Verification items for the finished model (mm, model axes). A direction names the side the tool comes from. Give positions to 0.01 mm unless a question says otherwise; leave off trailing zeros. Write item = value, one per line.
from build123d import *

# Parameters (mm, degrees)
SKETCH1_W                = 180
SKETCH1_H                = 180
SKETCH1_W_2              = 160
SKETCH1_H_2              = 160
SKETCH1_W_3              = 140
SKETCH1_H_3              = 140
BOSS_EXTRUDE1_DEPTH      = 3
SKETCH1_3_W              = 140
SKETCH1_3_H              = 140
BOSS_EXTRUDE2_DEPTH      = 5
SKETCH6_R                = 4.7
BOSS_EXTRUDE4_DEPTH      = 8
BOSS_EXTRUDE5_DEPTH      = 8
BOSS_EXTRUDE5_DRAFT      = 5
CUT_EXTRUDE1_START       = -5
SKETCH12_R               = 4.7
CUT_EXTRUDE1_DEPTH       = 5
SKETCH13_R               = 29.75
BOSS_EXTRUDE6_DEPTH      = 2.5
SKETCH14_R               = 29.75
SKETCH16_R               = 29.25
CUT_EXTRUDE2_START       = -2
CUT_EXTRUDE2_OUTLINE_R   = 34.25
CUT_EXTRUDE2_DEPTH       = 2
FILLET1_R                = 10
SKETCH19_W               = 140
SKETCH19_H               = 140
CUT_EXTRUDE3_DEPTH       = 5
F_5_16_CLEARANCE_HOLE1_D = 8.72998
SKETCH24_R               = 10
SKETCH24_R_2             = 4.36499
CUT_EXTRUDE4_DEPTH       = 7
CUT_EXTRUDE5_DEPTH       = 128.711589146


# Read off the part's stored shape, not the designer's step: CSK for M4 Flat Head Machine Screw1, Cut-Extrude2
with BuildPart() as part:
    # Sketch1 → Boss-Extrude1 (new body)
    # profile 1 of 3: a face of its own
    with BuildSketch(Plane(origin=(0, 0, 0), x_dir=(1, 0, 0), z_dir=(0, 1, 0))):
        Rectangle(SKETCH1_W, SKETCH1_H)
        Rectangle(SKETCH1_W_2, SKETCH1_H_2, mode=Mode.SUBTRACT)
    # profile 2 of 3: a face of its own
    with BuildSketch(Plane(origin=(0, 0, 0), x_dir=(1, 0, 0), z_dir=(0, 1, 0))):
        Rectangle(SKETCH1_W_2, SKETCH1_H_2)
        Rectangle(SKETCH1_W_3, SKETCH1_H_3, mode=Mode.SUBTRACT)
    # profile 3 of 3: a face of its own
    with BuildSketch(Plane(origin=(0, 0, 0), x_dir=(1, 0, 0), z_dir=(0, 1, 0))):
        Rectangle(SKETCH1_W_3, SKETCH1_H_3)
    extrude(amount=BOSS_EXTRUDE1_DEPTH)

    # Sketch1<3> → Boss-Extrude2 (add)
    with BuildSketch(Plane(origin=(0, 0, 0), x_dir=(1, 0, 0), z_dir=(0, 1, 0))):
        Rectangle(SKETCH1_3_W, SKETCH1_3_H)
    extrude(amount=-BOSS_EXTRUDE2_DEPTH)

    # CSK for M4 Flat Head Machine Screw1 outl → CSK for M4 Flat Head Machine Screw1 (revolve, cut)
    with BuildSketch(Plane(origin=(-80, 0, 0), x_dir=(1, 0, 0), z_dir=(0, 0, 1))):
        Polygon((0, 0), (2.4, 0), (2.4, 0.7), (4.7, 3), (0, 3), align=None)
    revolve(axis=Axis((-80, 0, 0), (0, 1, 0)), mode=Mode.SUBTRACT)

    # CSK for M4 Flat Head Machine Screw1 2 ou → CSK for M4 Flat Head Machine Screw1 2 (revolve, cut)
    with BuildSketch(Plane.XY.offset(80)):
        Polygon((0, 0), (2.4, 0), (2.4, 0.7), (4.7, 3), (0, 3), align=None)
    revolve(axis=Axis((0, 0, 80), (0, 1, 0)), mode=Mode.SUBTRACT)

    # CSK for M4 Flat Head Machine Screw1 3 ou → CSK for M4 Flat Head Machine Screw1 3 (revolve, cut)
    with BuildSketch(Plane(origin=(80, 0, 0), x_dir=(1, 0, 0), z_dir=(0, 0, 1))):
        Polygon((0, 0), (2.4, 0), (2.4, 0.7), (4.7, 3), (0, 3), align=None)
    revolve(axis=Axis((80, 0, 0), (0, 1, 0)), mode=Mode.SUBTRACT)

    # CSK for M4 Flat Head Machine Screw1 4 ou → CSK for M4 Flat Head Machine Screw1 4 (revolve, cut)
    with BuildSketch(Plane.XY.offset(-80)):
        Polygon((0, 0), (2.4, 0), (2.4, 0.7), (4.7, 3), (0, 3), align=None)
    revolve(axis=Axis((0, 0, -80), (0, 1, 0)), mode=Mode.SUBTRACT)

    # CSK for M4 Flat Head Machine Screw1 5 ou → CSK for M4 Flat Head Machine Screw1 5 (revolve, cut)
    with BuildSketch(Plane(origin=(-80, 0, 80), x_dir=(1, 0, 0), z_dir=(0, 0, 1))):
        Polygon((0, 0), (2.4, 0), (2.4, 0.7), (4.7, 3), (0, 3), align=None)
    revolve(axis=Axis((-80, 0, 80), (0, 1, 0)), mode=Mode.SUBTRACT)

    # CSK for M4 Flat Head Machine Screw1 6 ou → CSK for M4 Flat Head Machine Screw1 6 (revolve, cut)
    with BuildSketch(Plane(origin=(80, 0, -80), x_dir=(1, 0, 0), z_dir=(0, 0, 1))):
        Polygon((0, 0), (2.4, 0), (2.4, 0.7), (4.7, 3), (0, 3), align=None)
    revolve(axis=Axis((80, 0, -80), (0, 1, 0)), mode=Mode.SUBTRACT)

    # CSK for M4 Flat Head Machine Screw1 7 ou → CSK for M4 Flat Head Machine Screw1 7 (revolve, cut)
    with BuildSketch(Plane(origin=(80, 0, 80), x_dir=(1, 0, 0), z_dir=(0, 0, 1))):
        Polygon((0, 0), (2.4, 0), (2.4, 0.7), (4.7, 3), (0, 3), align=None)
    revolve(axis=Axis((80, 0, 80), (0, 1, 0)), mode=Mode.SUBTRACT)

    # CSK for M4 Flat Head Machine Screw1 8 ou → CSK for M4 Flat Head Machine Screw1 8 (revolve, cut)
    with BuildSketch(Plane(origin=(-80, 0, -80), x_dir=(1, 0, 0), z_dir=(0, 0, 1))):
        Polygon((0, 0), (2.4, 0), (2.4, 0.7), (4.7, 3), (0, 3), align=None)
    revolve(axis=Axis((-80, 0, -80), (0, 1, 0)), mode=Mode.SUBTRACT)

    # CSK for M4 Flat Head Machine Screw1 9 ou → CSK for M4 Flat Head Machine Screw1 9 (revolve, cut)
    with BuildSketch(Plane.XY):
        Polygon((0, -5), (2.4, -5), (2.4, 0.7), (4.7, 3), (0, 3), align=None)
    revolve(axis=Axis((0, 0, 0), (0, 1, 0)), mode=Mode.SUBTRACT)

    # Sketch6 → Boss-Extrude4 (add, through all)
    with BuildSketch(Plane(origin=(0, 3, 0), x_dir=(1, 0, 0), z_dir=(0, 1, 0))):
        with Locations(Location((80, 0, 0), (0, 0, 270))):
            Circle(SKETCH6_R)
        Circle(SKETCH6_R)
    extrude(amount=-BOSS_EXTRUDE4_DEPTH)


with BuildPart() as boss_extrude5_tool:
    # Sketch10 → Boss-Extrude5 (with draft: the straight prism first)
    with BuildSketch(Plane(origin=(0, 3, 0), x_dir=(1, 0, 0), z_dir=(0, 1, 0))):
        with BuildLine():
            Line((-70.393178849, -10), (-78.397496431, -10))
            ThreePointArc((-78.397496431, -10), (-76.604236916, -34.68045004), (-72.838821124, -59.137801445))
            ThreePointArc((-72.838821124, -59.137801445), (-52.739092363, -74.026279442), (-29.795427813, -83.98891616))
            ThreePointArc((-29.795427813, -83.98891616), (24.279800219, -59.374355653), (72.634248938, -24.851114715))
            ThreePointArc((72.634248938, -24.851114715), (75.478184725, 0), (72.634248938, 24.851114715))
            ThreePointArc((72.634248938, 24.851114715), (24.279800219, 59.374355653), (-29.795427813, 83.98891616))
            ThreePointArc((-29.795427813, 83.98891616), (-52.739092363, 74.026279442), (-72.838821124, 59.137801445))
            ThreePointArc((-72.838821124, 59.137801445), (-76.604236916, 34.68045004), (-78.397496431, 10))
            Line((-78.397496431, 10), (-70.393178849, 10))
            ThreePointArc((-70.393178849, 10), (-68.785863401, 32.603044383), (-65.480018889, 55.020726474))
            ThreePointArc((-65.480018889, 55.020726474), (-48.739092363, 67.098076211), (-29.909337417, 75.557468997))
            ThreePointArc((-29.909337417, 75.557468997), (20.279800219, 52.446152423), (65.389356306, 20.536742523))
            ThreePointArc((65.389356306, 20.536742523), (67.478184725, 0), (65.389356306, -20.536742523))
            ThreePointArc((65.389356306, -20.536742523), (20.279800219, -52.446152423), (-29.909337417, -75.557468997))
            ThreePointArc((-29.909337417, -75.557468997), (-48.739092363, -67.098076211), (-65.480018889, -55.020726474))
            ThreePointArc((-65.480018889, -55.020726474), (-68.785863401, -32.603044383), (-70.393178849, -10))
        make_face()
    extrude(amount=BOSS_EXTRUDE5_DEPTH)
    # Boss-Extrude5: the draft: its side faces are tilted about the plane it starts from
    boss_extrude5_sides = [boss_extrude5_tool.faces().sort_by_distance(p)[0] for p in [
        (-74.39533764, 7, 10),
        (-76.604236916, 7, 34.68045004),
        (-52.739092363, 7, 74.026279442),
        (24.279800219, 7, 59.374355653),
        (75.478184725, 7, 0),
        (24.279800219, 7, -59.374355653),
        (-52.739092363, 7, -74.026279442),
        (-76.604236916, 7, -34.68045004),
        (-74.39533764, 7, -10),
        (-68.785863401, 7, -32.603044383),
        (-48.739092363, 7, -67.098076211),
        (20.279800219, 7, -52.446152423),
        (67.478184725, 7, 0),
        (20.279800219, 7, 52.446152423),
        (-48.739092363, 7, 67.098076211),
        (-68.785863401, 7, 32.603044383),
    ]]
    draft(boss_extrude5_sides, Plane(origin=(0, 3, 0), x_dir=(1, 0, 0), z_dir=(0, 1, 0)), BOSS_EXTRUDE5_DRAFT)


with BuildPart() as part_1:
    add(part.part)

    # Boss-Extrude5: add boss_extrude5_tool
    add(boss_extrude5_tool.part)

    # Sketch12 → Cut-Extrude1 (cut)
    with BuildSketch(Plane.XZ.offset(5).offset(CUT_EXTRUDE1_START)):
        with Locations((80, 0)):
            Circle(SKETCH12_R)
    extrude(amount=CUT_EXTRUDE1_DEPTH, mode=Mode.SUBTRACT)

    # Sketch13 → Boss-Extrude6 (add)
    with BuildSketch(Plane(origin=(0, 3, 0), x_dir=(1, 0, 0), z_dir=(0, 1, 0))):
        with Locations(Location((-10, 0, 0), (0, 0, 270))):
            Circle(SKETCH13_R)
    extrude(amount=BOSS_EXTRUDE6_DEPTH)

    # Sketch14 → Loft1 section 0
    with BuildSketch(Plane(origin=(0, 5.5, 0), x_dir=(1, 0, 0), z_dir=(0, 1, 0))):
        with Locations((-10, 0)):
            Circle(SKETCH14_R)
    # Sketch16 → Loft1 section 1
    with BuildSketch(Plane(origin=(0, 15.5, 0), x_dir=(1, 0, 0), z_dir=(0, 1, 0))):
        with Locations((-10, 0)):
            Circle(SKETCH16_R)
    loft()

    # Cut-Extrude2 outline → Cut-Extrude2 (cut)
    with BuildSketch(Plane(origin=(0, 15.5, 0), x_dir=(1, 0, 0), z_dir=(0, 1, 0)).offset(CUT_EXTRUDE2_START)):
        with Locations((-10, 0)):
            Circle(CUT_EXTRUDE2_OUTLINE_R)
    extrude(amount=CUT_EXTRUDE2_DEPTH, mode=Mode.SUBTRACT)

    # Fillet1
    fillet1_edges = [part_1.edges().sort_by_distance(p)[0] for p in [
        (-90, 1.5, 90),
        (-90, 1.5, -90),
        (90, 1.5, -90),
        (90, 1.5, 90),
    ]]
    fillet(fillet1_edges, radius=FILLET1_R)

    # Sketch19 → Cut-Extrude3 (cut)
    with BuildSketch(Plane.XZ.offset(5)):
        Rectangle(SKETCH19_W, SKETCH19_H)
    extrude(amount=-CUT_EXTRUDE3_DEPTH, mode=Mode.SUBTRACT)

    # 5/16 Clearance Hole1 (through all)
    with Locations(Plane(origin=(0, 13.5, 0), x_dir=(1, 0, 0), z_dir=(0, 1, 0))):
        with Locations((-18.75, 15.155444566), (7.5, 0), (-18.75, -15.155444566)):
            Hole(F_5_16_CLEARANCE_HOLE1_D / 2)

    # Sketch24 → Cut-Extrude4 (cut)
    # profile 1 of 6: a face of its own
    with BuildSketch(Plane.XZ):
        with Locations(Location((-18.75, 15.155444566, 0), (0, 0, 270))):
            Circle(SKETCH24_R)
        with Locations(Location((-18.75, 15.155444566, 0), (0, 0, 90))):
            Circle(SKETCH24_R_2, mode=Mode.SUBTRACT)
    # profile 2 of 6: a face of its own
    with BuildSketch(Plane.XZ):
        with Locations(Location((7.5, 0, 0), (0, 0, 270))):
            Circle(SKETCH24_R)
        with Locations(Location((7.5, 0, 0), (0, 0, 90))):
            Circle(SKETCH24_R_2, mode=Mode.SUBTRACT)
    # profile 3 of 6: a face of its own
    with BuildSketch(Plane.XZ):
        with Locations(Location((-18.75, -15.155444566, 0), (0, 0, 270))):
            Circle(SKETCH24_R)
        with Locations(Location((-18.75, -15.155444566, 0), (0, 0, 90))):
            Circle(SKETCH24_R_2, mode=Mode.SUBTRACT)
    # profile 4 of 6: a face of its own
    with BuildSketch(Plane.XZ):
        with Locations(Location((-18.75, -15.155444566, 0), (0, 0, 90))):
            Circle(SKETCH24_R_2)
    # profile 5 of 6: a face of its own
    with BuildSketch(Plane.XZ):
        with Locations(Location((-18.75, 15.155444566, 0), (0, 0, 90))):
            Circle(SKETCH24_R_2)
    # profile 6 of 6: a face of its own
    with BuildSketch(Plane.XZ):
        with Locations(Location((7.5, 0, 0), (0, 0, 90))):
            Circle(SKETCH24_R_2)
    extrude(amount=-CUT_EXTRUDE4_DEPTH, mode=Mode.SUBTRACT)

    # Sketch25 → Cut-Extrude5 (cut, through all)
    with BuildSketch(Plane(origin=(0, 3, 0), x_dir=(1, 0, 0), z_dir=(0, 1, 0))):
        with BuildLine():
            Line((90, -80), (90, 80))
            ThreePointArc((90, 80), (87.071067812, 87.071067812), (80, 90))
            Line((80, 90), (-80, 90))
            ThreePointArc((-80, 90), (-87.071067812, 87.071067812), (-90, 80))
            Line((-90, 80), (-90, -80))
            ThreePointArc((-90, -80), (-87.071067812, -87.071067812), (-80, -90))
            Line((-80, -90), (80, -90))
            ThreePointArc((80, -90), (87.071067812, -87.071067812), (90, -80))
        make_face()
        with BuildLine():
            Line((-80, 89.8), (80, 89.8))
            ThreePointArc((80, 89.8), (86.929646456, 86.929646456), (89.8, 80))
            Line((89.8, 80), (89.8, -80))
            ThreePointArc((89.8, -80), (86.929646456, -86.929646456), (80, -89.8))
            Line((80, -89.8), (-80, -89.8))
            ThreePointArc((-80, -89.8), (-86.929646456, -86.929646456), (-89.8, -80))
            Line((-89.8, -80), (-89.8, 80))
            ThreePointArc((-89.8, 80), (-86.929646456, 86.929646456), (-80, 89.8))
        make_face(mode=Mode.SUBTRACT)
    extrude(amount=-CUT_EXTRUDE5_DEPTH, mode=Mode.SUBTRACT)


solid = part_1.part
1) Material ranges on probe 1 along X at (y, z) = (0.55, 80); probe 2 along Z at (x, y) = (80, 0.2), recorded low to high. Write a range as from..to.
From the geometry:
probe_1 = -89.8..-82.4, -77.6..-2.4, 2.4..77.6, 82.4..89.8
probe_2 = -89.8..-82.4, -77.6..77.6, 82.4..89.8
2) Draft check along X on faces 1 (the cylindrical face through (-86.85, 1.52, 87.01)), 2 (the cylindrical face through (-0.31, 0.35, -82.38)), 3 (the conical face through (75.133, 6.944, 0.35)). Enter one of: +X half, -X half, draft (parallel to the pull), parting line (faces both ways), or undercut.
From the geometry:
face_1 = -X half
face_2 = undercut
face_3 = +X half
3) Tool access check on faces 4 (the cylindrical face through (-10.32, 3.45, 9.78)), 5 (the conical face through (19.78, 6.94, -53.13)), 6 (the flat face through (-74.339, 6.944, 10.345)). Record the directions out of +Z, -Z, +X, -X, +Y, -Y that give a thin tool (end or side, any length) a straight path to the whole face; none if there is none.
From the geometry:
face_4 = -Y
face_5 = +Y
face_6 = -X, +Y
4) Cross-section at A-A on x = -18.75. Count the separate pieces of the cut face and the enclosed holes in it, plus the area to 3 significant figures.
From the geometry:
separate_pieces = 3
enclosed_holes = 0
area = 865 mm^2
5) Depth check by flat-ended pin: P1, Ø6, axis at x = 6.5, z = -4, coming from the -Y side; P2, Ø7, axis at x = -18.75, z = -15.16, coming from the -Y side; P3, Ø8, axis at x = -23, y = 8, coming from the -Z side; P4, Ø1.5, axis at x = -19.5, y = 4.5, coming from the -Z side. Enter the tip coordinate at first touch or a pass-through.
From the geometry:
P1 = 7
P2 = through
P3 = -82.6
P4 = -80.4
